For this review, take the finished solid that the model builds, in its own axes (mm). Face numbers are marked on the shaded views. A direction names the side the tool comes from. Give positions to 0.01 mm unless a question says otherwise; leave off trailing zeros. Write each loop counter-clockwise with the first axis right and the second up, starting at its lowest first coordinate (ties: lowest second). Pieces come first, ordered by that corner, then holes.
Q1. We need section D-D (y = -13). Write out the cut boundary in (x, z).
Q2. Insertion check: P1, Ø1, axis at y = 17.5, z = 13, coming from the -X side; P2, Ø0.5, axis at x = -17, z = 15.5, coming from the +Y side; P3, Ø0.6, axis at y = -17.5, z = 8, coming from the -X side; P4, Ø12, axis at x = -15.5, y = -13, coming from the -Z side. Each pin has a flat end and moves straight along its axis. Give the tip position at first contact, or say it passes through.
Q3. We need section A-A (y = 15). Write out the cut boundary in (x, z).
Q4. Machinability: for the marked faces 1, 2, 3 and 4, which of the approach directions +Z, -Z, +X, -X, +Y, -Y give a long, thin tool a straight path to every point of the face, cutting with its end or side? Answer none if there is none.
Q5. We need section B-B (y = -4.5). Write out the cut boundary in (x, z).
Q6. We need section C-C (x = 2). Write out the cut boundary in (y, z).
Q7. Mouldability with a two-part tool opening along X and no side actions: class the marked faces 5, 6 and 7 as released by +X, released by -X, zero draft, split by the parting line, or undercut.
Q8. For line 1 (X direction, y = -14.5, z = 23.5); line 2 (Y direction, x = 4.5, z = 16.75); line 3 (Y direction, x = 6, z = 8), list the stretches that pass through material, from the lowest coordinate up.
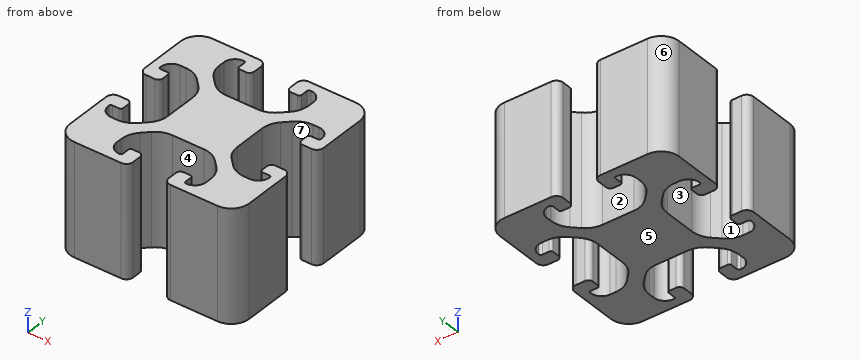
```python
from build123d import *

# Parameters (mm, degrees)
F1_DEPTH = 25


with BuildPart() as f1:
    # F0 (on Top) → F1 (new body)
    with BuildSketch(Plane.XY):
        with BuildLine():
            Line((-16.5, -4), (-18.5, -4))
            ThreePointArc((-18.5, -4), (-19.56066, -4.43934), (-20, -5.5))
            Line((-20, -5.5), (-20, -16))
            ThreePointArc((-20, -16), (-18.828427, -18.828427), (-16, -20))
            Line((-16, -20), (-5.5, -20))
            ThreePointArc((-5.5, -20), (-4.43934, -19.56066), (-4, -18.5))
            Line((-4, -18.5), (-4, -16.5))
            ThreePointArc((-4, -16.5), (-4.292893, -15.792893), (-5, -15.5))
            Line((-5, -15.5), (-6.5, -15.5))
            ThreePointArc((-6.5, -15.5), (-6.853553, -15.646447), (-7, -16))
            Line((-7, -16), (-7, -17.55))
            ThreePointArc((-7, -17.55), (-7.131802, -17.868198), (-7.45, -18))
            Line((-7.45, -18), (-7.5, -18))
            ThreePointArc((-7.5, -18), (-9.267767, -17.267767), (-10, -15.5))
            Line((-10, -15.5), (-10, -14.192388))
            ThreePointArc((-10, -14.192388), (-9.619398, -12.278971), (-8.535534, -10.656854))
            Line((-8.535534, -10.656854), (-7.093146, -9.214466))
            ThreePointArc((-7.093146, -9.214466), (-5.471029, -8.130602), (-3.557612, -7.75))
            Line((-3.557612, -7.75), (3.557612, -7.75))
            ThreePointArc((3.557612, -7.75), (5.471029, -8.130602), (7.093146, -9.214466))
            Line((7.093146, -9.214466), (8.535534, -10.656854))
            ThreePointArc((8.535534, -10.656854), (9.619398, -12.278971), (10, -14.192388))
            Line((10, -14.192388), (10, -15.5))
            ThreePointArc((10, -15.5), (9.267767, -17.267767), (7.5, -18))
            Line((7.5, -18), (7.45, -18))
            ThreePointArc((7.45, -18), (7.131802, -17.868198), (7, -17.55))
            Line((7, -17.55), (7, -16))
            ThreePointArc((7, -16), (6.853553, -15.646447), (6.5, -15.5))
            Line((6.5, -15.5), (5, -15.5))
            ThreePointArc((5, -15.5), (4.292893, -15.792893), (4, -16.5))
            Line((4, -16.5), (4, -18.5))
            ThreePointArc((4, -18.5), (4.43934, -19.56066), (5.5, -20))
            Line((5.5, -20), (16, -20))
            ThreePointArc((16, -20), (18.828427, -18.828427), (20, -16))
            Line((20, -16), (20, -5.5))
            ThreePointArc((20, -5.5), (19.56066, -4.43934), (18.5, -4))
            Line((18.5, -4), (16.5, -4))
            ThreePointArc((16.5, -4), (15.792893, -4.292893), (15.5, -5))
            Line((15.5, -5), (15.5, -6.5))
            ThreePointArc((15.5, -6.5), (15.646447, -6.853553), (16, -7))
            Line((16, -7), (17.55, -7))
            ThreePointArc((17.55, -7), (17.868198, -7.131802), (18, -7.45))
            Line((18, -7.45), (18, -7.5))
            ThreePointArc((18, -7.5), (17.267767, -9.267767), (15.5, -10))
            Line((15.5, -10), (14.192388, -10))
            ThreePointArc((14.192388, -10), (12.278971, -9.619398), (10.656854, -8.535534))
            Line((10.656854, -8.535534), (9.214466, -7.093146))
            ThreePointArc((9.214466, -7.093146), (8.130602, -5.471029), (7.75, -3.557612))
            Line((7.75, -3.557612), (7.75, 3.557612))
            ThreePointArc((7.75, 3.557612), (8.130602, 5.471029), (9.214466, 7.093146))
            Line((9.214466, 7.093146), (10.656854, 8.535534))
            ThreePointArc((10.656854, 8.535534), (12.278971, 9.619398), (14.192388, 10))
            Line((14.192388, 10), (15.5, 10))
            ThreePointArc((15.5, 10), (17.267767, 9.267767), (18, 7.5))
            Line((18, 7.5), (18, 7.45))
            ThreePointArc((18, 7.45), (17.868198, 7.131802), (17.55, 7))
            Line((17.55, 7), (16, 7))
            ThreePointArc((16, 7), (15.646447, 6.853553), (15.5, 6.5))
            Line((15.5, 6.5), (15.5, 5))
            ThreePointArc((15.5, 5), (15.792893, 4.292893), (16.5, 4))
            Line((16.5, 4), (18.5, 4))
            ThreePointArc((18.5, 4), (19.56066, 4.43934), (20, 5.5))
            Line((20, 5.5), (20, 16))
            ThreePointArc((20, 16), (18.828427, 18.828427), (16, 20))
            Line((16, 20), (5.5, 20))
            ThreePointArc((5.5, 20), (4.43934, 19.56066), (4, 18.5))
            Line((4, 18.5), (4, 16.5))
            ThreePointArc((4, 16.5), (4.292893, 15.792893), (5, 15.5))
            Line((5, 15.5), (6.5, 15.5))
            ThreePointArc((6.5, 15.5), (6.853553, 15.646447), (7, 16))
            Line((7, 16), (7, 17.55))
            ThreePointArc((7, 17.55), (7.131802, 17.868198), (7.45, 18))
            Line((7.45, 18), (7.5, 18))
            ThreePointArc((7.5, 18), (9.267767, 17.267767), (10, 15.5))
            Line((10, 15.5), (10, 14.192388))
            ThreePointArc((10, 14.192388), (9.619398, 12.278971), (8.535534, 10.656854))
            Line((8.535534, 10.656854), (7.093146, 9.214466))
            ThreePointArc((7.093146, 9.214466), (5.471029, 8.130602), (3.557612, 7.75))
            Line((3.557612, 7.75), (-3.557612, 7.75))
            ThreePointArc((-3.557612, 7.75), (-5.471029, 8.130602), (-7.093146, 9.214466))
            Line((-7.093146, 9.214466), (-8.535534, 10.656854))
            ThreePointArc((-8.535534, 10.656854), (-9.619398, 12.278971), (-10, 14.192388))
            Line((-10, 14.192388), (-10, 15.5))
            ThreePointArc((-10, 15.5), (-9.267767, 17.267767), (-7.5, 18))
            Line((-7.5, 18), (-7.45, 18))
            ThreePointArc((-7.45, 18), (-7.131802, 17.868198), (-7, 17.55))
            Line((-7, 17.55), (-7, 16))
            ThreePointArc((-7, 16), (-6.853553, 15.646447), (-6.5, 15.5))
            Line((-6.5, 15.5), (-5, 15.5))
            ThreePointArc((-5, 15.5), (-4.292893, 15.792893), (-4, 16.5))
            Line((-4, 16.5), (-4, 18.5))
            ThreePointArc((-4, 18.5), (-4.43934, 19.56066), (-5.5, 20))
            Line((-5.5, 20), (-16, 20))
            ThreePointArc((-16, 20), (-18.828427, 18.828427), (-20, 16))
            Line((-20, 16), (-20, 5.5))
            ThreePointArc((-20, 5.5), (-19.56066, 4.43934), (-18.5, 4))
            Line((-18.5, 4), (-16.5, 4))
            ThreePointArc((-16.5, 4), (-15.792893, 4.292893), (-15.5, 5))
            Line((-15.5, 5), (-15.5, 6.5))
            ThreePointArc((-15.5, 6.5), (-15.646447, 6.853553), (-16, 7))
            Line((-16, 7), (-17.55, 7))
            ThreePointArc((-17.55, 7), (-17.868198, 7.131802), (-18, 7.45))
            Line((-18, 7.45), (-18, 7.5))
            ThreePointArc((-18, 7.5), (-17.267767, 9.267767), (-15.5, 10))
            Line((-15.5, 10), (-14.192388, 10))
            ThreePointArc((-14.192388, 10), (-12.278971, 9.619398), (-10.656854, 8.535534))
            Line((-10.656854, 8.535534), (-9.214466, 7.093146))
            ThreePointArc((-9.214466, 7.093146), (-8.130602, 5.471029), (-7.75, 3.557612))
            Line((-7.75, 3.557612), (-7.75, -3.557612))
            ThreePointArc((-7.75, -3.557612), (-8.130602, -5.471029), (-9.214466, -7.093146))
            Line((-9.214466, -7.093146), (-10.656854, -8.535534))
            ThreePointArc((-10.656854, -8.535534), (-12.278971, -9.619398), (-14.192388, -10))
            Line((-14.192388, -10), (-15.5, -10))
            ThreePointArc((-15.5, -10), (-17.267767, -9.267767), (-18, -7.5))
            Line((-18, -7.5), (-18, -7.45))
            ThreePointArc((-18, -7.45), (-17.868198, -7.131802), (-17.55, -7))
            Line((-17.55, -7), (-16, -7))
            ThreePointArc((-16, -7), (-15.646447, -6.853553), (-15.5, -6.5))
            Line((-15.5, -6.5), (-15.5, -5))
            ThreePointArc((-15.5, -5), (-15.792893, -4.292893), (-16.5, -4))
        make_face()
    extrude(amount=F1_DEPTH)


solid = f1.part
```
Computed:
1. outline: (-20, 0) - (-9.86, 0) - (-9.86, 25) - (-20, 25) - close; (9.86, 0) - (20, 0) - (20, 25) - (9.86, 25) - close
2. P1: stops at x = -19.87
2. P2: stops at y = 19.93
2. P3: stops at x = -19.82
2. P4: stops at z = 0
3. outline: (-20, 0) - (-10, 0) - (-10, 25) - (-20, 25) - close; (10, 0) - (20, 0) - (20, 25) - (10, 25) - close
4. face 1: +Z, -Z
4. face 2: +Z, -Z, +Y
4. face 3: +Z, -Z, -X
4. face 4: +Z, -Z, -Y
5. outline: (-19.62, 0) - (-15.63, 0) - (-15.63, 25) - (-19.62, 25) - close; (-7.84, 0) - (7.84, 0) - (7.84, 25) - (-7.84, 25) - close; (15.63, 0) - (19.62, 0) - (19.62, 25) - (15.63, 25) - close
6. outline: (-7.75, 0) - (7.75, 0) - (7.75, 25) - (-7.75, 25) - close
7. face 5: zero draft
7. face 6: released by -X
7. face 7: undercut
8. line 1: x = -20 to -10, 10 to 20
8. line 2: y = -19.62 to -15.63, -7.84 to 7.84, 15.63 to 19.62
8. line 3: y = -20 to -15.5, -8.39 to 8.39, 15.5 to 20
